Autodesk Inventor part; units mm, degrees
ref_plane "Plano de trabalho1" through (171, -3, -14) normal (0, 0, -1) x (-1, 0, 0)
ref_plane "YZ Plane" through (0, 0, 0) normal (1, 0, 0) x (0, 1, 0)
ref_plane "XZ Plane" through (0, 0, 0) normal (0, 1, 0) x (-1, 0, 0)
sketch "Esboço1" plane through (0, 0, 0) normal (0, 1, 0) x (-1, 0, 0)
  line L0 (-133, -3) -> (0, -3)
  line L1 (0, -25) -> (-98, -25)
  line L2 (-133, 0) -> (-133, -28)
  line L3 (-133, -28) -> (-123, -28)
  line L4 (-95, -28) -> (0, -28)
  line L5 (0, -28) -> (0, 0)
  line L6 (0, 0) -> (-133, 0)
  line L7 (-95, -28) -> (-95, -53)
  line L8 (-95, -53) -> (-133, -53)
  line L9 (-133, -53) -> (-133, -50)
  line L10 (-133, -50) -> (-98, -50)
  line L11 (-98, -50) -> (-98, -25)
  arc A0 (-123, -50) -> (-98, -25) centre (-123, -25) ccw
  arc A1 (-123, -28) -> (-120, -25) centre (-123, -25) ccw
  line L12 (-133, -25) -> (-120, -25)
  line L13 (0, 0) -> (3, 0)
  line L14 (3, 0) -> (3, -28)
  line L15 (3, -28) -> (0, -28)
  line L16 (-123, -28) -> (-123, -25)
  line L17 (-133, -50) -> (-133, -28)
  line L18 (0, -3) -> (3, -3)
  line L19 (0, -25) -> (3, -25)
  line L20 (-133, -3) -> (-266, -3)
  line L21 (-266, -25) -> (-168, -25)
  line L22 (-133, -28) -> (-143, -28)
  line L23 (-171, -28) -> (-266, -28)
  line L24 (-266, -28) -> (-266, 0)
  line L25 (-266, 0) -> (-133, 0)
  line L26 (-171, -28) -> (-171, -53)
  line L27 (-171, -53) -> (-133, -53)
  line L28 (-133, -50) -> (-168, -50)
  line L29 (-168, -50) -> (-168, -25)
  arc A2 (-168, -25) -> (-143, -50) centre (-143, -25) ccw
  arc A3 (-146, -25) -> (-143, -28) centre (-143, -25) ccw
  line L30 (-133, -25) -> (-146, -25)
  line L31 (-266, 0) -> (-269, 0)
  line L32 (-269, 0) -> (-269, -28)
  line L33 (-269, -28) -> (-266, -28)
  line L34 (-143, -28) -> (-143, -25)
  line L35 (-266, -3) -> (-269, -3)
  line L36 (-266, -25) -> (-269, -25)
  point P0 (-133, -14)
  point P1 (-133, -51.5)
  point P2 (-83, -28)
  dimension "d7" = 22
  dimension "d9" = 3
  dimension "d10" = 3
  dimension "d13" = 3
  dimension "d14" = 3
  dimension "d16" = 22
  dimension "d20" = 22
  dimension "d21" = 120
  dimension "d29" = 3
  dimension "d31" = 10
extrude "Extrusão1" add sketch "Esboço1" against normal blind 3 contours L20 L24 L25 L2 | L2 L30 A3 L22 L17 L28 A2 L21 L24 L20 | L2 L22 L34 L30 | L35 L32 L31 L24 | L24 L36 L32 L35 | L34 A3 L30 | L21 L29 L28 L9 L27 L26 L23 L24 | L24 L33 L32 L36 | A2 L28 L29
extrude "Extrusão2" add sketch "Esboço1" along normal blind 10 contours L20 L24 L25 L2 | L2 L22 L34 L30 | L35 L32 L31 L24 | L21 L29 L28 L9 L27 L26 L23 L24 | L24 L33 L32 L36
sketch "Esboço2" plane through (133, -3, 0) normal (0, 0, 1) x (1, 0, 0)
  line L0 (0, 13) -> (136, 13)
  line L1 (136, 0) -> (0, 0)
  line L2 (136, 0) -> (155.9239, 1.7431)
  line L3 (136, 0) -> (156, 0) construction
  line L4 (155.9239, 1.7431) -> (154.7952, 14.6444)
  line L5 (154.7952, 14.6444) -> (136, 13)
  line L6 (136, 0) -> (136, 13)
  line L7 (136, 0) -> (136, 13)
  dimension "d32" = 20
  dimension "d33" = 5
extrude "Extrusão4" add sketch "Esboço2" against normal up to surface (28 mm away)
ref_plane "Plano de trabalho1" through (171, -3, -14) normal (0, 0, -1) x (-1, 0, 0)
sketch "Esboço3" plane through (171, -3, -14) normal (0, 0, -1) x (-1, 0, 0)
  line L0 (-116.7952, 14.6444) -> (-98, 13)
  line L1 (3, 13) -> (-98, 13)
  line L2 (-98, 0) -> (-117.9239, 1.7431)
  line L3 (-117.6667, 4.6824) -> (-98.4366, 3)
  line L4 (-98.4366, 3) -> (-98, 3)
  line L5 (-117.9239, 1.7431) -> (-116.7952, 14.6444)
  line L6 (-117.6667, 4.6824) -> (-116.7952, 14.6444)
  line L7 (-116.7952, 14.6444) -> (-98, 13)
  line L8 (-98, 13) -> (-98, 3)
  dimension "d36" = 10
extrude "Extrusão5" cut sketch "Esboço3" along normal mid plane 22
equation "\"d9\" = mdf"
equation "\"d10\" = mdf"
equation "\"d13\" = mdf"
equation "\"d14\" = mdf"
equation "\"mdf\" = 3"
equation "\"margem\" = 1"
properties part number "Trilho 5 min"
Could you check a few things on this model? Use its own coordinates, in mm. A direction names the side the tool comes from. Round coordinates to 2 decimals unless told otherwise and drop trailing zeros. Loops run counter-clockwise (first coordinate to the right, second up) from the corner with the lowest first, then second, coordinate; pieces in that order, holes last. Notation, with made-up numbers: (-25, 50.5) -> (-6, 50.5) arc R20 ccw to (-6, 82.5) -> close; hole circle Ø2 at (36.25, 21.25). An arc over 180 degrees is marked (long way). Put each result on its own line as item: value.
Q1. I want a section at C-C on z = -22.5. Write out the boundary of the cut face in (x, y), and give its area (3 significant figures).
Checks:
outline: (133, -3) -> (269, -3) -> (288.92, -1.26) -> (288.67, 1.68) -> (269.44, 0) -> (133, 0) -> close
area: 467 mm2
Q2. For pin 1 Ø7.5 at (x, y) = (255, 0.5) entering from -Z; pin 2 Ø2 at (y, z) = (9.5, -40.5) entering from +X; pin 3 Ø4 at (y, z) = (9, -43.5) entering from -X, each with a flat end and sliding along its axis, tell me the tip position at first contact or that it passes through.
Checks:
pin 1: z = -28
pin 2: x = 171
pin 3: x = 168
Q3. Thinking about a two-plate mould opening in Z: for faces 6 (the flat face through (210, 3, 0)), 7 (the flat face through (229, 4, -28)), 8 (the flat face through (187, 0, -16)), which applies, pulls with the +Z half, pulls with the -Z half, needs draft (parallel to the pull), parting line crosses it, or undercut?
Checks:
face 6: pulls with the +Z half
face 7: pulls with the -Z half
face 8: undercut
Q4. I want a section at D-D on x = 191. Write out the boundary of the cut face in (y, z), and give its area (3 significant figures).
Checks:
outline: (-3, -28) -> (10, -28) -> (10, -25) -> (0, -25) -> (0, -3) -> (10, -3) -> (10, 0) -> (-3, 0) -> close
area: 144 mm2
Q5. I want a section at A-A on x = 157. Write out the boundary of the cut face in (y, z).
Checks:
outline: (-3, -53) -> (10, -53) -> (10, -50) -> (0, -50) -> (0, -3) -> (10, -3) -> (10, 0) -> (-3, 0) -> close
Q6. I want a section at B-B on y = 7. Write out the boundary of the cut face in (x, z).
Checks:
outline: (133, -53) -> (171, -53) -> (171, -28) -> (288.2, -28) -> (288.2, -25) -> (168, -25) -> (168, -50) -> (133, -50) -> close; (133, -28) -> (143, -28) -> (143, -25) -> (133, -25) -> close; (133, -3) -> (288.2, -3) -> (288.2, 0) -> (133, 0) -> close
Q7. Please list where these lines run through material, in increasing order: line 1 (Z direction, x = 155, y = 6.5); line 2 (Z direction, x = 217, y = 9.5); line 3 (Z direction, x = 141.5, y = 6). Write a range as from..to.
Checks:
line 1: -53..-50, -3..0
line 2: -28..-25, -3..0
line 3: -53..-50, -28..-25, -3..0
Q8. Which directions (+Z, -Z, +X, -X, +Y, -Y) give clear straight access to the entire face, cutting with the end or side of a thin tool? Please do faces 1 (the flat face through (288.744, 0.803, -13.804)), 2 (the flat face through (150, 5, -50)), 3 (the flat face through (138, 10, -26)), 4 (the flat face through (143, 5, -27)), 5 (the flat face through (171, 4, -40)).
Checks:
face 1: +Z, -Z, +X, +Y
face 2: -X, +Y
face 3: +Z, -Z, -X, +Y
face 4: +Y
face 5: -Z, +X, +Y, -Y
